Design review of the part shown in the three views and the two pictorial views. Dimensions are in mm from the part's minimum x, y and z. Give positions to 0.01 mm unless a question says otherwise; leave off trailing zeros. Loops run counter-clockwise (first coordinate to the right, second up) from the corner with the lowest first, then second, coordinate; pieces in that order, holes last. Notation, with made-up numbers: (54.25, 33.25) - (64.25, 33.25) arc R25 cw to (64.25, 62.25) - close; hole circle Ø7 at (-15.5, 82). An arc over 180 degrees is marked (long way). Use CSV: the item, a comma, the result in double quotes. Start each with the question number.
1. Wall thickness on line 1 (X direction, y = 2.5, z = 74.5) (1 decimal); line 2 (Z direction, x = 2.05, y = 0.65); line 3 (X direction, y = 2.45, z = 50) (1 decimal): over which ranges is each line inside the solid? List them lowest first.
2. Take a section at A-A on z = 55.5. Give the boundary of the cut face in (x, y).
3. For pin 1 (1.5 mm diameter, centred on y = 3, z = 50, fed in from +X); pin 2 (2 mm diameter, centred on x = 2.89, y = 2.5, fed in from +Z), all flat-tipped, find the tip position at first contact; note any pin that passes through.
4. Take a section at B-B on x = 0.7. Give the boundary of the cut face in (y, z).
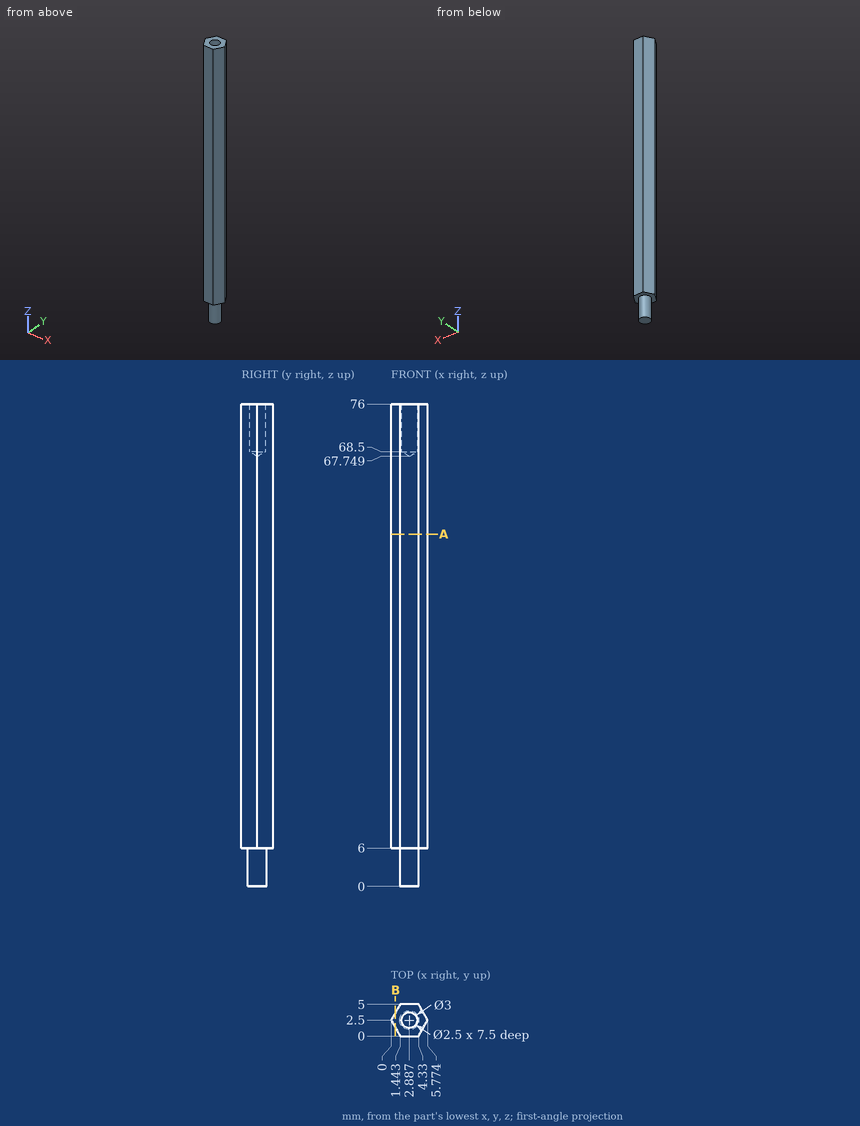
Check result:
1,line 1,"x = 0 to 1.6, 4.1 to 5.8"
1,line 2,"z = 6 to 76"
1,line 3,"x = 0 to 5.7"
2,outline,"(0, 2.5) - (1.44, 0) - (4.33, 0) - (5.77, 2.5) - (4.33, 5) - (1.44, 5) - close"
3,pin 1,"stops at x = 5.77"
3,pin 2,"stops at z = 68.35"
4,outline,"(1.29, 6) - (3.71, 6) - (3.71, 76) - (1.29, 76) - close"
